Verification items for the finished model (mm, model axes). Face numbers are marked on the shaded views. A direction names the side the tool comes from. Give positions to 0.01 mm unless a question says otherwise; leave off trailing zeros. One line per item, written item: value. Start each with the question number.
1. Scan lines: L1, parallel to Z at x = -139, y = 84 (3 decimals); L2, parallel to Y at x = 150, z = 23 (3 decimals); L3, parallel to Y at x = -23, z = 17. Record each from-to range of solid material in increasing order. Write a range as [from, to].
2. Gauge pin test, flat ends, axial feed: pin 1 (12.5 mm diameter, centred on y = -76, z = 33.5, fed in from +X) (3 decimals); pin 2 (2.5 mm diameter, centred on y = -161.5, z = 17.5, fed in from +X); pin 3 (17.5 mm diameter, centred on y = 143, z = 29, fed in from -X). Record the tip position at first contact, or that the pin passes through.
3. Access from +Z, -Z, +X, -X, +Y, -Y to the whole of each face (thin tool, end or side, straight path). Record for the marked faces 1 and 2.
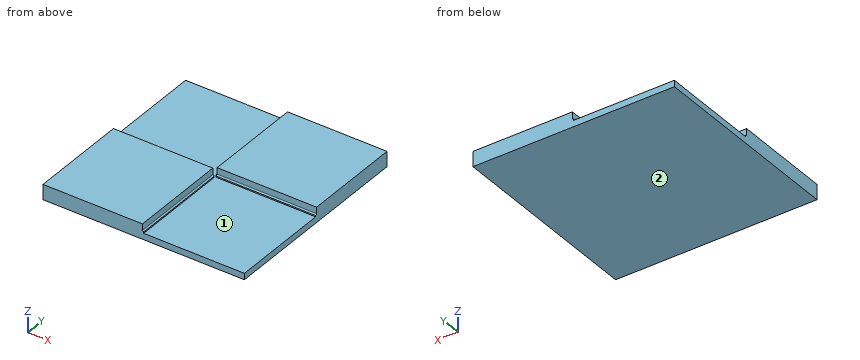
from build123d import *

# Parameters (mm, degrees)
F0_W     = 508
F0_H     = 508
F1_DEPTH = 38.1
F2_W     = 250.825
F2_H     = 250.825
F2_H_2   = 6.35
F2_W_2   = 6.35
F3_DEPTH = 19.05
F4_R     = 3.17499
F6_DEPTH = 22.225


# Not quite as in the source:
# - a fillet or chamfer is up to 0.001 mm smaller than in the source, because OpenCascade refuses the exact size
# - a pattern or mirror of a feature is missing from the dataset's text; its kind, count and spacing are read off the source's solid


with BuildPart() as f1:
    # F0 (on Top) → F1 (new body)
    with BuildSketch(Plane.XY):
        Rectangle(F0_W, F0_H)
    extrude(amount=F1_DEPTH)

    # F2 (on face) → F3 (cut)
    with BuildSketch(Plane.XY.offset(38.1)):
        with Locations((128.5875, -128.5875)):
            Rectangle(F2_W, F2_H)
        with Locations((128.5875, 0)):
            Rectangle(F2_W, F2_H_2)
        with Locations((0, -128.5875)):
            Rectangle(F2_W_2, F2_H)
        Rectangle(F2_W_2, F2_H_2)
        with Locations((-128.5875, 0)):
            Rectangle(F2_W, F2_H_2)
        with Locations((0, 128.5875)):
            Rectangle(F2_W_2, F2_H)
    extrude(amount=-F3_DEPTH, mode=Mode.SUBTRACT)

    # F4 (radius 3.175 in the source; OpenCascade refuses exactly that, so slightly less here)
    f4_edges = [f1.edges().sort_by_distance(p)[0] for p in [
        (-128.5875, -3.175, 19.05),
        (-3.175, -128.5875, 19.05),
        (3.175, 128.5875, 19.05),
        (128.5875, 3.175, 19.05),
        (-3.175, 128.5875, 19.05),
        (-128.5875, 3.175, 19.05),
    ]]
    fillet(f4_edges, radius=F4_R)

    # F5 (on face) → F6 (cut)
    with BuildSketch(Plane.XY.offset(38.1)):
        Polygon((0, 254), (-254, 254), (-254, 0), (-3.3675960454, 0), (-1.6837980227, -1.6837980227), (1.6837980227, 1.6837980227), (0, 3.3675960454), align=None)
    f6 = extrude(amount=-F6_DEPTH, mode=Mode.SUBTRACT)

    # F6_copies: F6 across plane
    add(f6.mirror(Plane(origin=(0, 0, 0), x_dir=(-0.7071067812, -0.7071067812, 0), z_dir=(0.7071067812, -0.7071067812, 0))), mode=Mode.SUBTRACT)


solid = f1.part
Results are:
1. L1: z = [0, 15.875]
1. L2: y = [3.175, 254]
1. L3: y = [-254, 0]
2. pin 1: stops at x = -3.175
2. pin 2: stops at x = 0
2. pin 3: stops at x = 2.49
3. face 1: +Z
3. face 2: -Z, +X, -X, +Y, -Y
